For this review, use the dimensioned drawing (mm, ordinates from the lowest corner) and the shaded views. A direction names the side the tool comes from. Coordinates: 2 decimals unless noted, no trailing zeros. Write each loop counter-clockwise with the first axis right and the second up, starting at its lowest first coordinate (ties: lowest second). Pieces come first, ordered by that corner, then holes. Notation, with made-up numbers: (59, 74) - (103, 74) arc R21 ccw to (103, 104) - close; hole circle Ø7 at (-37.75, 46). An arc over 180 degrees is marked (long way). Use one line per item in the form item = value. Start each with the question number.
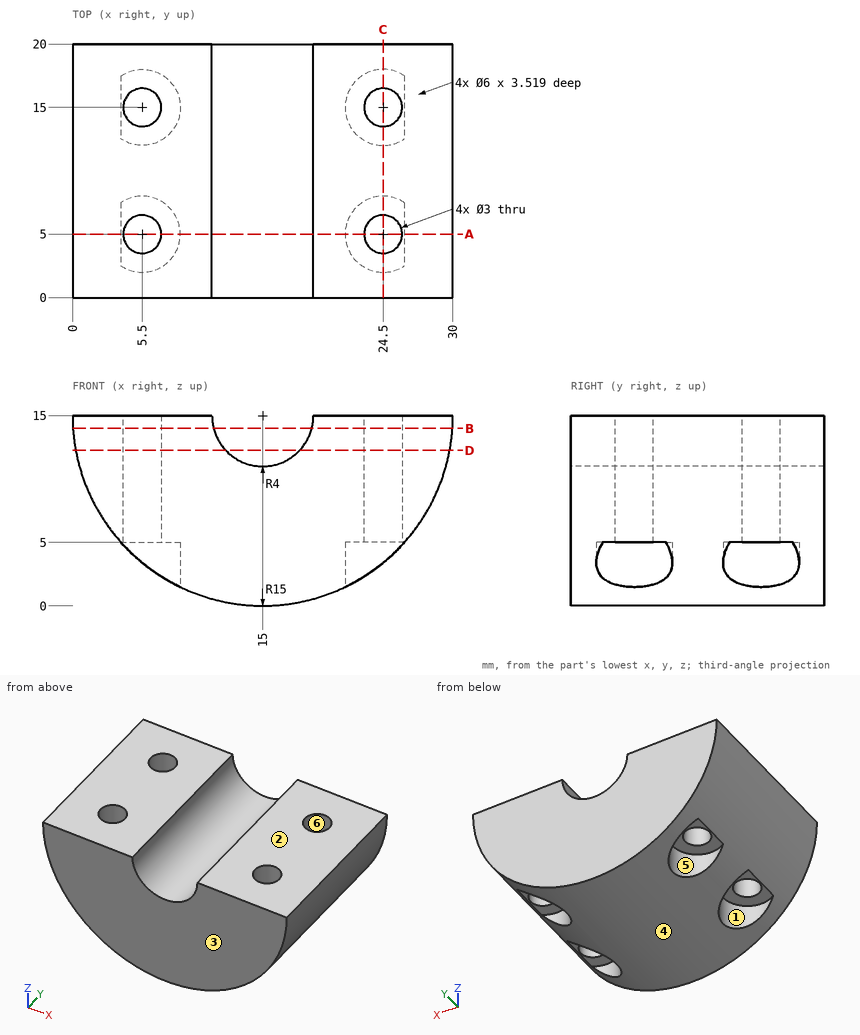
1. The part is to be moulded in two halves that separate along X. For the marked faces 3, 4, 5 and 6, say which applies: released by +X, released by -X, zero draft, split by the parting line, or undercut.
2. Take a section at B-B (z = 14). State the section outline as (x, y) points.
3. For P1, Ø1.4, axis at x = 6.5, y = 5, coming from the -Z side; P2, Ø4, axis at y = 9.5, z = 3, coming from the +X side; P3, Ø7, axis at x = 5.5, y = 5, coming from the -Z side; P4, Ø2.5, axis at x = 24.5, y = 5, coming from the +Z side, all flat-tipped, find the tip position at first contact; note any pin that passes through.
4. For the marked faces 1 and 2, list the 3-axis set-ups (+Z, -Z, +X, -X, +Y, -Y) from which the entire face can be reached by the end or side of a thin tool; tool diameter is ignored.
5. Take a section at D-D (z = 12.25). State the section outline as (x, y) points (1 decimal).
6. For L1, parallel to Y at x = 24.5, z = 11.5; L2, parallel to X at y = 15.25, z = 12.5 (1 decimal); L3, parallel to Y at x = 24, z = 3.75, list the stretches that pass through material, from the lowest coordinate up.
7. Take a section at C-C (x = 24.5). State the section outline as (y, z) points.
8. Take a section at A-A (y = 5). State the section outline as (x, z) points.
Returned:
q1.face_3 = zero draft
q1.face_4 = split by the parting line
q1.face_5 = undercut
q1.face_6 = undercut
q2.outline = (0.03, 0) - (11.13, 0) - (11.13, 20) - (0.03, 20) - close; (18.87, 0) - (29.97, 0) - (29.97, 20) - (18.87, 20) - close; hole circle Ø3 at (5.5, 5); hole circle Ø3 at (5.5, 15); hole circle Ø3 at (24.5, 5); hole circle Ø3 at (24.5, 15)
q3.P1 = 5
q3.P2 = 26.18
q3.P3 = 1.25
q3.P4 = through
q4.face_1 = -Z
q4.face_2 = +Z, +X, -X, +Y, -Y
q5.outline = (0.3, 0) - (12.1, 0) - (12.1, 20) - (0.3, 20) - close; (17.9, 0) - (29.7, 0) - (29.7, 20) - (17.9, 20) - close; hole circle Ø3 at (5.5, 5); hole circle Ø3 at (5.5, 15); hole circle Ø3 at (24.5, 5); hole circle Ø3 at (24.5, 15)
q6.L1 = 0 to 3.5, 6.5 to 13.5, 16.5 to 20
q6.L2 = 0.2 to 4, 7 to 11.9, 18.1 to 23, 26 to 29.8
q6.L3 = 0 to 2.04, 7.96 to 12.04, 17.96 to 20
q7.outline = (0, 3.39) - (2, 3.39) - (2, 5) - (3.5, 5) - (3.5, 15) - (0, 15) - close; (6.5, 5) - (8, 5) - (8, 3.39) - (12, 3.39) - (12, 5) - (13.5, 5) - (13.5, 15) - (6.5, 15) - close; (16.5, 5) - (18, 5) - (18, 3.39) - (20, 3.39) - (20, 15) - (16.5, 15) - close
q8.outline = (0, 15) arc R15 ccw to (3.82, 5) - (4, 5) - (4, 15) - close; (7, 5) - (8.5, 5) - (8.5, 1.48) arc R15 ccw to (21.5, 1.48) - (21.5, 5) - (23, 5) - (23, 15) - (19, 15) arc R4 cw to (11, 15) - (7, 15) - close; (26, 5) - (26.18, 5) arc R15 ccw to (30, 15) - (26, 15) - close
